```python
from build123d import *

# Parameters (mm, degrees)
BASE_FLANGE1_DEPTH = 1613
CUT_EXTRUDE1_REACH = 1615.878
FILLET1_R          = 3
CUT_EXTRUDE2_REACH = 1615.878
SKETCH7_R          = 4.5
LPATTERN1_COUNT    = 4
LPATTERN1_PITCH    = 529


# Sheet-metal steps are written as plain solids
with BuildPart() as part:
    # Sketch1 → Base-Flange1 (new body)
    with BuildSketch(Plane(origin=(0, 0, 0), x_dir=(1, 0, 0), z_dir=(0, 1, 0))):
        with BuildLine():
            Line((-25, 25), (-25, 4.5))
            ThreePointArc((-25, 4.5), (-23.681980515, 1.318019485), (-20.5, 0))
            Line((-20.5, 0), (20.5, 0))
            ThreePointArc((20.5, 0), (23.681980515, 1.318019485), (25, 4.5))
            Line((25, 4.5), (25, 25))
            Line((25, 25), (22, 25))
            Line((22, 25), (22, 4.5))
            ThreePointArc((22, 4.5), (21.560660172, 3.439339828), (20.5, 3))
            Line((20.5, 3), (-20.5, 3))
            ThreePointArc((-20.5, 3), (-21.560660172, 3.439339828), (-22, 4.5))
            Line((-22, 4.5), (-22, 25))
            Line((-22, 25), (-25, 25))
        make_face()
    extrude(amount=BASE_FLANGE1_DEPTH)

    # Sketch6 → Cut-Extrude1 (cut, up to next)
    with BuildSketch(Plane(origin=(-22, 0, 0), x_dir=(0, 0, -1), z_dir=(1, 0, 0)), mode=Mode.PRIVATE) as cut_extrude1_sk1:
        with BuildLine():
            Line((12.5, 18), (18.5, 18))
            ThreePointArc((18.5, 18), (23.5, 13), (18.5, 8))
            Line((18.5, 8), (12.5, 8))
            ThreePointArc((12.5, 8), (7.5, 13), (12.5, 18))
        make_face()
    cut_extrude1_tool1 = extrude(cut_extrude1_sk1.sketch, amount=-CUT_EXTRUDE1_REACH, mode=Mode.PRIVATE) & part.part
    cut_extrude1 = cut_extrude1_tool1.solids().sort_by_distance((-22, 13, -15.5))[0]
    add(cut_extrude1, mode=Mode.SUBTRACT)

    # Fillet1
    fillet1_edges = [part.edges().sort_by_distance(p)[0] for p in [
        (23.5, 0, -25),
        (-23.5, 0, -25),
        (23.5, 1613, -25),
        (-23.5, 1613, -25),
    ]]
    fillet(fillet1_edges, radius=FILLET1_R)

    # Sketch7 → Cut-Extrude2 (cut, up to next)
    with BuildSketch(Plane.ZY.offset(-22), mode=Mode.PRIVATE) as cut_extrude2_sk1:
        with Locations((-15.5, 13)):
            Circle(SKETCH7_R)
    cut_extrude2_tool1 = extrude(cut_extrude2_sk1.sketch, amount=-CUT_EXTRUDE2_REACH, mode=Mode.PRIVATE) & part.part
    cut_extrude2 = cut_extrude2_tool1.solids().sort_by_distance((22, 13, -15.5))[0]
    add(cut_extrude2, mode=Mode.SUBTRACT)

    # LPattern1: Cut-Extrude1, Cut-Extrude2 ×4
    with Locations(*[(0, i * LPATTERN1_PITCH, 0) for i in range(1, LPATTERN1_COUNT)]):
        add(cut_extrude1, mode=Mode.SUBTRACT)
        add(cut_extrude2, mode=Mode.SUBTRACT)


solid = part.part
```
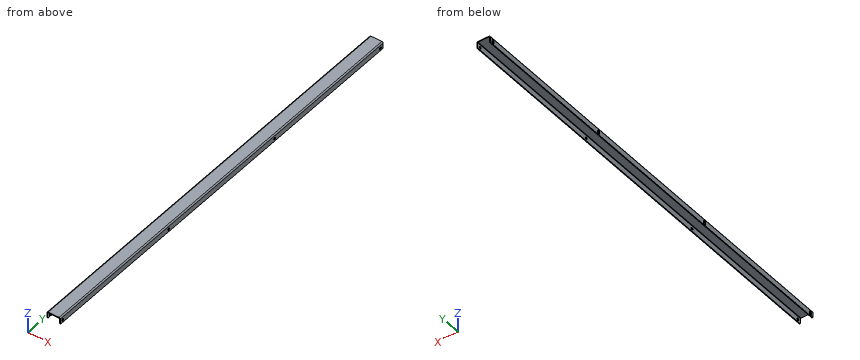
Part model, mm, in its own coordinate system. Give positions to 0.01 mm unless a question says otherwise; leave off trailing zeros. Write each loop counter-clockwise with the first axis right and the second up, starting at its lowest first coordinate (ties: lowest second). Pieces come first, ordered by that corner, then holes. Notation, with made-up numbers: (56.25, 73) -> (88.25, 73) arc R37 cw to (88.25, 111) -> close; hole circle Ø3 at (12, 86). An arc over 180 degrees is marked (long way). Put each result on its own line as item: value. Start each with the question number.
Item 1: Pin check, flat tip, straight feed: pin 1 Ø5 at (x, y) = (8, 919) entering from -Z. Stop position of the tip, or through.
Item 2: Cut at A-A (y = 974.5). List the corners of the cut face in (x, z).
Item 3: Cut at B-B (x = 6). List the corners of the cut face in (y, z).
Item 4: Wall check: L1, parallel to Y at x = 24, z = -15.5; L2, parallel to X at y = 390, z = -3.75; L3, parallel to X at y = 1152, z = -11.25. Give the ranges that are in metal, low to high. Write a range as [from, to].
Answer list:
1. pin 1: stops at z = -3
2. outline: (-25, -25) -> (-22, -25) -> (-22, -4.5) arc R1.5 cw to (-20.5, -3) -> (20.5, -3) arc R1.5 cw to (22, -4.5) -> (22, -25) -> (25, -25) -> (25, -4.5) arc R4.5 ccw to (20.5, 0) -> (-20.5, 0) arc R4.5 ccw to (-25, -4.5) -> close
3. outline: (0, -3) -> (1613, -3) -> (1613, 0) -> (0, 0) -> close
4. L1: y = [0, 8.5], [17.5, 537.5], [546.5, 1066.5], [1075.5, 1595.5], [1604.5, 1613]
4. L2: x = [-24.94, -21.8], [21.8, 24.94]
4. L3: x = [-25, -22], [22, 25]
